Solid Edge part; units mm, degrees
sketch "Sketch1" plane through (0, 0, 0) normal (0, -1, 0) x (1, 0, 0)
  line L0 (0, 15) -> (0, -15)
  line L1 (0, -15) -> (30, -15)
  line L2 (30, -15) -> (30, -13)
  line L3 (30, -13) -> (2, -13)
  line L4 (2, -13) -> (2, 13)
  line L5 (2, 13) -> (30, 13)
  line L6 (30, 13) -> (30, 15)
  line L7 (30, 15) -> (0, 15)
  dimension "D1" = 30
  dimension "D2" = 30
extrude "Protrusion1" add sketch "Sketch1" along normal mid plane 200
sketch "Sketch2" plane through (15, 0, 15) normal (0, 0, 1) x (0, -1, 0)
  line L0 (0, 15) -> (0, -5)
  line L1 (0, -5) -> (100, -5)
  line L2 (100, -5) -> (100, 15)
  line L3 (100, 15) -> (0, 15)
  dimension "D1" = 100
extrude "Cutout1" cut sketch "Sketch2" against normal through all
hole "Hole_1" at (2, -87.5, 0) direction (-1, 0, 0) diameter 5 end up to next
hole "Hole1" at (2, -12.5, 0) direction (-1, 0, 0) diameter 5 end up to next
hole "Hole_3" at (17.5, 95, -15) direction (0, 0, 1) diameter 4.8 end through all
hole "Hole2" at (17.5, 75, -15) direction (0, 0, 1) diameter 4.8 end through all
properties material "Aluminum, 1060"
Input: part model. Units: mm. Frame: model coordinates. A direction names the side the tool comes from. Give positions to 0.01 mm unless a question says otherwise; leave off trailing zeros. Loops run counter-clockwise (first coordinate to the right, second up) from the corner with the lowest first, then second, coordinate; pieces in that order, holes last. Notation, with made-up numbers: (22.25, 26.5) -> (38.25, 26.5) arc R23 cw to (38.25, 35.5) -> close; hole circle Ø8 at (-21, -29). An arc over 180 degrees is marked (long way). Answer as a JSON object with one key per item and string values. Group by question number.
Item 1: Line query: probe 1 along Y at (x, z) = (17.5, -13.45); probe 2 along X at (y, z) = (95, 13.9); probe 3 along Z at (x, y) = (25, 4). Output: solid intervals per line, ascending.
Item 2: Reachability of faces 5 (the flat face through (13, 24, -13)), 6 (the cylindrical face through (16.581, 77.217, -14.014)) from +Z, -Z, +X, -X, +Y, -Y: full face, straight path, thin tool, end or side. Return the list, or none.
Item 3: Cut plane B-B, the plane y = -87.5. Return the cut outline in (x, z).
Item 4: Pull-direction query (X, two-part tool) for faces 1 (the flat face through (0, 1, 0)), 2 (the cylindrical face through (16.581, 77.217, 13.986)), 3 (the flat face through (13, 24, 13)), 4 (the flat face through (2, 1, 0)); classes: released by +X, released by -X, zero draft, split by the parting line, or undercut.
Item 5: Cut plane C-C, the plane z = 0. Return the cut outline in (x, y), and give its area (3 significant figures).
Item 6: Pin query (flat end, axial travel): P1, Ø10, axis at y = -36, z = -4.5, coming from the -X side; P2, Ø4.5, axis at y = -12.5, z = 0, coming from the -X side; P3, Ø2, axis at y = -31, z = -14.5, coming from the +X side; P4, Ø8, axis at y = 1, z = 6, coming from the +X side. Return the tip coordinate at first contact, or that it passes through.
Item 7: Cut plane A-A, the plane x = 8. Return the cut outline in (y, z), and give its area (3 significant figures).
Item 8: Cut plane D-D, the plane y = 75. Return the cut outline in (x, z), and give its area (3 significant figures).
Checks:
{
 "1": {"probe 1": "y = 0 to 72.6, 77.4 to 92.6, 97.4 to 100", "probe 2": "x = 0 to 15.1, 19.9 to 30", "probe 3": "z = -15 to -13, 13 to 15"},
 "2": {"face 5": "+X, +Y, -Y", "face 6": "+Z, -Z"},
 "3": {"outline": "(0, -15) -> (10, -15) -> (10, -13) -> (2, -13) -> (2, -2.5) -> (0, -2.5) -> close; (0, 2.5) -> (2, 2.5) -> (2, 13) -> (10, 13) -> (10, 15) -> (0, 15) -> close"},
 "4": {"face 1": "released by -X", "face 2": "undercut", "face 3": "zero draft", "face 4": "released by +X"},
 "5": {"outline": "(0, -100) -> (2, -100) -> (2, -90) -> (0, -90) -> close; (0, -85) -> (2, -85) -> (2, -15) -> (0, -15) -> close; (0, -10) -> (2, -10) -> (2, 100) -> (0, 100) -> close", "area": "380 mm²"},
 "6": {"P1": "stops at x = 0", "P2": "passes through", "P3": "stops at x = 10", "P4": "stops at x = 2"},
 "7": {"outline": "(-100, -15) -> (100, -15) -> (100, -13) -> (-100, -13) -> close; (-100, 13) -> (100, 13) -> (100, 15) -> (-100, 15) -> close", "area": "800 mm²"},
 "8": {"outline": "(0, -15) -> (15.1, -15) -> (15.1, -13) -> (2, -13) -> (2, 13) -> (15.1, 13) -> (15.1, 15) -> (0, 15) -> close; (19.9, -15) -> (30, -15) -> (30, -13) -> (19.9, -13) -> close; (19.9, 13) -> (30, 13) -> (30, 15) -> (19.9, 15) -> close", "area": "153 mm²"}
}
